The listing builds one solid part. Answer for the finished solid, in the listing's coordinates (mm). A direction names the side the tool comes from. Give positions to 0.01 mm unless a question says otherwise; leave off trailing zeros. Write each loop counter-clockwise with the first axis right and the second up, starting at its lowest first coordinate (ties: lowest second). Pieces come first, ordered by that corner, then holes. Notation, with made-up numbers: (-39.75, 53) - (18.25, 53) arc R16 ccw to (18.25, 80) - close; hole circle Ø2 at (-40, 70.25). An arc over 180 degrees is marked (long way). Answer as CSV lines item,"result". Start each with the question number.
(1) Find section C-C (y = 0.85). State how many separate pieces and enclosed holes the cut face has, then the cut area to 3 significant figures.
(2) For a pull along X with two mould halves and no side action, classify faces 4 (the face through (100, 1, -81)), 5 (the face through (66, 1, -93)), 6 (the face through (2, 1, -87)), 7 (the face through (5, 1, 15)) as pulls with the +X half, pulls with the -X half, needs draft (parallel to the pull), parting line crosses it, or undercut.
(3) Each of these flat-tipped pins is pushed along its axis until it touches: pin 1 Ø1.5 at (y, z) = (1.5, -93) entering from -X; pin 2 Ø0.9 at (y, z) = (1.5, -93.5) entering from +X; pin 3 Ø0.9 at (y, z) = (1, 28) entering from +X. Where does it stop, or does it pass through?
(4) Straight lines are drawn through the part: probe 1 along X at (y, z) = (0.8, -43.5); probe 2 along X at (y, z) = (1.05, -31.6); probe 3 along Z at (x, y) = (66.5, 0.6). For each, find the intervals that lie inside material, in ascending order.
(5) For faces 1 (the face through (54, 1, -94)), 2 (the face through (1, 1, -35)), 3 (the face through (97, 1, -71)), determine the directions among +Z, -Z, +X, -X, +Y, -Y from which every point of the face is accessible in a straight line to the end or side of a thin tool.
(6) Find section B-B (z = -31.6). Write down the section's boundary in (x, y).
(7) Find section A-A (x = 30). Write down the section's boundary in (y, z), then the cut area to 3 significant figures.
from build123d import *

# Parameters (mm, degrees)
ESQUISSE1_R        = 2.05
ESQUISSE1_R_2      = 1.5
BOSS_EXTRU_1_DEPTH = 3


with BuildPart() as part:
    # Esquisse1 → Boss.-Extru.1 (new body)
    with BuildSketch(Plane(origin=(0, 0, 0), x_dir=(1, 0, 0), z_dir=(0, 1, 0))):
        Polygon((44, -30), (56, -30), (56, -27), (64, -27), (64, -30), (76, -30), (76, -27), (84, -27), (84, -30), (90, -30), (100, 0), (100, 7), (97, 7), (97, 15), (100, 15), (100, 27), (97, 27), (97, 35), (100, 35), (100, 47), (97, 47), (97, 55), (100, 55), (100, 67), (97, 67), (97, 75), (100, 75), (100, 87), (97, 87), (97, 95), (94, 95), (94, 92), (86, 92), (86, 95), (74, 95), (74, 92), (66, 92), (66, 95), (54, 95), (54, 92), (46, 92), (46, 95), (34, 95), (34, 92), (26, 92), (26, 95), (14, 95), (14, 92), (6, 92), (6, 95), (3, 95), (3, 87), (0, 87), (0, 75), (3, 75), (3, 67), (0, 67), (0, 55), (3, 55), (3, 47), (0, 47), (0, 35), (3, 35), (3, 27), (0, 27), (0, 15), (3, 15), (3, 7), (0, 7), (0, 0), (10, -30), (16, -30), (16, -27), (24, -27), (24, -30), (36, -30), (36, -27), (44, -27), align=None)
        with Locations(Location((66.05, 0.55, 0), (0, 0, 270))):
            Circle(ESQUISSE1_R, mode=Mode.SUBTRACT)
        with Locations(Location((38.05, 0.55, 0), (0, 0, 270))):
            Circle(ESQUISSE1_R, mode=Mode.SUBTRACT)
        with Locations(Location((38.05, -22.95, 0), (0, 0, 270))):
            Circle(ESQUISSE1_R, mode=Mode.SUBTRACT)
        with Locations(Location((66.05, -22.95, 0), (0, 0, 270))):
            Circle(ESQUISSE1_R, mode=Mode.SUBTRACT)
        with Locations(Location((30, 80, 0), (0, 0, 270))):
            Circle(ESQUISSE1_R_2, mode=Mode.SUBTRACT)
        with Locations(Location((30, 43.5, 0), (0, 0, 270))):
            Circle(ESQUISSE1_R_2, mode=Mode.SUBTRACT)
        with Locations(Location((11.604719745, 8.5, 0), (0, 0, 270))):
            Circle(ESQUISSE1_R_2, mode=Mode.SUBTRACT)
        with Locations(Location((11.604719745, 31.6, 0), (0, 0, 270))):
            Circle(ESQUISSE1_R_2, mode=Mode.SUBTRACT)
        with Locations(Location((58.504719745, 31.6, 0), (0, 0, 270))):
            Circle(ESQUISSE1_R_2, mode=Mode.SUBTRACT)
        with Locations(Location((66.5, 80, 0), (0, 0, 270))):
            Circle(ESQUISSE1_R_2, mode=Mode.SUBTRACT)
        with Locations(Location((66.5, 43.5, 0), (0, 0, 270))):
            Circle(ESQUISSE1_R_2, mode=Mode.SUBTRACT)
        with Locations(Location((58.504719745, 8.5, 0), (0, 0, 270))):
            Circle(ESQUISSE1_R_2, mode=Mode.SUBTRACT)
    extrude(amount=BOSS_EXTRU_1_DEPTH)


solid = part.part
Result set:
1,separate pieces,"1"
1,enclosed holes,"12"
1,area,"11,600 mm^2"
2,face 4,"pulls with the +X half"
2,face 5,"undercut"
2,face 6,"needs draft"
2,face 7,"pulls with the -X half"
3,pin 1,"x = 3"
3,pin 2,"x = 97"
3,pin 3,"x = 90.82"
4,probe 1,"0 to 28.5, 31.5 to 65, 68 to 100"
4,probe 2,"3 to 10.1, 13.1 to 57, 60 to 97"
4,probe 3,"-92 to -81.5, -78.5 to -45, -42 to -2.55, 1.45 to 20.95, 24.95 to 30"
5,face 1,"-Z, +Y, -Y"
5,face 2,"-X, +Y, -Y"
5,face 3,"+X, +Y, -Y"
6,outline,"(3, 0) - (10.1, 0) - (10.1, 3) - (3, 3) - close; (13.1, 0) - (57, 0) - (57, 3) - (13.1, 3) - close; (60, 0) - (97, 0) - (97, 3) - (60, 3) - close"
7,outline,"(0, -92) - (3, -92) - (3, -81.5) - (0, -81.5) - close; (0, -78.5) - (3, -78.5) - (3, -45) - (0, -45) - close; (0, -42) - (3, -42) - (3, 30) - (0, 30) - close"
7,area,"348 mm^2"
